Geometry: final body of the model. Coordinates: model frame, mm. A direction names the side the tool comes from. Give positions to 0.01 mm unless a question says otherwise; leave off trailing zeros. Loops run counter-clockwise (first coordinate to the right, second up) from the corner with the lowest first, then second, coordinate; pieces in that order, holes last. Notation, with made-up numbers: (69.5, 64.25) -> (110.5, 64.25) arc R22 cw to (110.5, 70.25) -> close; hole circle Ø11 at (18, -26). An arc over 180 degrees is marked (long way). One line per question, with ' | ' between items. Start each with the question number.
Item 1: Material intervals for line 1 along Y through (x, z) = (-0.5, 842); line 2 along Z through (x, y) = (-52, 28); line 3 along X through (y, z) = (-25, 111), sorted ascending. Write a range as [from, to].
Item 2: Section C-C on z = 342.5. Return loops of the section in (x, y), then the cut area to 3 significant figures.
Item 3: Mould query, pull axis Y, two halves, no side actions, for faces 3 (the flat face through (-1, 1, 8)), 4 (the cylindrical face through (42.445, 13.367, 501)), 5 (the flat face through (-41, 19, 1008)), 6 (the flat face through (-99.55, -98.44, 3.94)). Classes: released by +Y, released by -Y, zero draft, split by the parting line, or undercut.
Item 4: Pin query (flat end, axial travel): P1, Ø2, axis at x = -45.5, z = 762, coming from the -Y side; P2, Ø1, axis at y = 39, z = 605.5, coming from the -X side; P3, Ø1.5, axis at y = 25, z = 179.5, coming from the -X side. Return the tip coordinate at first contact, or that it passes through.
Item 5: Section A-A on y = 0. Return loops of the section in (x, z), then the cut area to 3 significant figures.
Item 6: Set-up query: faces 1 (the flat face through (-98.44, 99.55, 3.94)), 2 (the cylindrical face through (-6.44, 49.08, 501)). Return all of +Z, -Z, +X, -X, +Y, -Y with unobstructed straight access to the full face (end or side cutting, diameter ignored); none if empty.
Item 7: Section D-D on y = -97. Return loops of the section in (x, z), then the cut area to 3 significant figures.
Item 8: Section B-B on x = 13. Return loops of the section in (y, z), then the cut area to 3 significant figures.
from build123d import *

# Parameters (mm, degrees)
F1_DEPTH = 8
F2_R     = 49.5
F2_R_2   = 44.500001
F3_DEPTH = 1000
F4_R     = 5


with BuildPart() as f1:
    # F0 (on Top) → F1 (new body)
    with BuildSketch(Plane.XY):
        Polygon((57.989899, 140), (-57.989899, 140), (-140, 57.989899), (-140, -57.989899), (-57.989899, -140), (57.989899, -140), (140, -57.989899), (140, 57.989899), align=None)
    extrude(amount=F1_DEPTH)

    # F2 (on face) → F3 (join)
    with BuildSketch(Plane.XY.offset(8)):
        Circle(F2_R)
        Circle(F2_R_2, mode=Mode.SUBTRACT)
    extrude(amount=F3_DEPTH)

    # F4
    f4_edges = [f1.edges().sort_by_distance(p)[0] for p in [
        (57.989899, 140, 4),
        (-57.989899, 140, 4),
        (-140, 57.989899, 4),
        (-140, -57.989899, 4),
        (-57.989899, -140, 4),
        (57.989899, -140, 4),
        (140, -57.989899, 4),
        (140, 57.989899, 4),
    ]]
    fillet(f4_edges, radius=F4_R)


solid = f1.part
Result sheet:
1) line 1: y = [-49.5, -44.5], [44.5, 49.5] | line 2: z = [0, 8] | line 3: x = [-42.72, -36.81], [36.81, 42.72]
2) outline: circle Ø99 at (0, 0); hole circle Ø89 at (0, 0) | area: 1,480 mm²
3) face 3: undercut | face 4: undercut | face 5: zero draft | face 6: released by -Y
4) P1: stops at y = -21.68 | P2: stops at x = -31.11 | P3: stops at x = -43.15
5) outline: (-140, 0) -> (140, 0) -> (140, 8) -> (49.5, 8) -> (49.5, 1008) -> (44.5, 1008) -> (44.5, 8) -> (-44.5, 8) -> (-44.5, 1008) -> (-49.5, 1008) -> (-49.5, 8) -> (-140, 8) -> close | area: 12,200 mm²
6) face 1: +Z, -Z, -X, +Y | face 2: +Z
7) outline: (-100.99, 0) -> (100.99, 0) -> (100.99, 8) -> (-100.99, 8) -> close | area: 1,620 mm²
8) outline: (-140, 0) -> (140, 0) -> (140, 8) -> (47.76, 8) -> (47.76, 1008) -> (42.56, 1008) -> (42.56, 8) -> (-42.56, 8) -> (-42.56, 1008) -> (-47.76, 1008) -> (-47.76, 8) -> (-140, 8) -> close | area: 12,600 mm²
